from build123d import *

# Parameters (mm, degrees)
SKETCH1_W           = 23.2
SKETCH1_H           = 12.1
BOSS_EXTRUDE1_DEPTH = 21.6
BOSS_EXTRUDE2_DEPTH = 1.8
SKETCH5_R           = 6.05
BOSS_EXTRUDE3_DEPTH = 3.9
SKETCH6_R           = 2.345
BOSS_EXTRUDE4_DEPTH = 3.1
SKETCH7_W           = 3.926136304
SKETCH7_H           = 5.6
BOSS_EXTRUDE5_DEPTH = 3.3


with BuildPart() as part:
    # Sketch1 → Boss-Extrude1 (new body)
    with BuildSketch(Plane(origin=(0, 0, 0), x_dir=(1, 0, 0), z_dir=(0, 1, 0))):
        Rectangle(SKETCH1_W, SKETCH1_H)
    extrude(amount=BOSS_EXTRUDE1_DEPTH)

    # Sketch3 → Boss-Extrude2 (add)
    with BuildSketch(Plane(origin=(0, 15.5, 0), x_dir=(-1, 0, 0), z_dir=(0, -1, 0))):
        with BuildLine():
            Line((-11.6, 2.8e-08), (-11.6, 6.05))
            Line((-11.6, 6.05), (-16.1, 6.05))
            Line((-16.1, 6.05), (-16.1, 1.6))
            ThreePointArc((-16.1, 1.6), (-13.285381067, 2.387990792), (-11.6, 2.8e-08))
        make_face()
        with BuildLine():
            Line((-11.6, -6.05), (-11.6, 2.8e-08))
            ThreePointArc((-11.6, 2.8e-08), (-13.28538104, -2.387990782), (-16.1, -1.6))
            Line((-16.1, -1.6), (-16.1, -6.05))
            Line((-16.1, -6.05), (-11.6, -6.05))
        make_face()
        with BuildLine():
            ThreePointArc((16.1, -1.6), (13.285381054, -2.387990787), (11.6, -1e-09))
            Line((11.6, -1e-09), (11.6, -6.05))
            Line((11.6, -6.05), (16.1, -6.05))
            Line((16.1, -6.05), (16.1, -1.6))
        make_face()
        with BuildLine():
            Line((16.1, 1.6), (16.1, 6.05))
            Line((16.1, 6.05), (11.6, 6.05))
            Line((11.6, 6.05), (11.6, -1e-09))
            ThreePointArc((11.6, -1e-09), (13.285381053, 2.387990787), (16.1, 1.6))
        make_face()
    extrude(amount=-BOSS_EXTRUDE2_DEPTH)

    # Sketch5 → Boss-Extrude3 (add)
    with BuildSketch(Plane(origin=(0, 21.6, 0), x_dir=(1, 0, 0), z_dir=(0, 1, 0))):
        with Locations((5.55, 0)):
            Circle(SKETCH5_R)
    extrude(amount=BOSS_EXTRUDE3_DEPTH)

    # Sketch6 → Boss-Extrude4 (add)
    with BuildSketch(Plane(origin=(0, 25.5, 0), x_dir=(1, 0, 0), z_dir=(0, 1, 0))):
        with Locations((5.55, 0)):
            Circle(SKETCH6_R)
    extrude(amount=BOSS_EXTRUDE4_DEPTH)

    # Sketch7 → Boss-Extrude5 (add)
    with BuildSketch(Plane(origin=(0, 21.6, 0), x_dir=(1, 0, 0), z_dir=(0, 1, 0))):
        with Locations((-0.95, 0)):
            Rectangle(SKETCH7_W, SKETCH7_H)
    extrude(amount=BOSS_EXTRUDE5_DEPTH)


solid = part.part
Input: part model. Units: mm. Frame: model coordinates. A direction names the side the tool comes from. Give positions to 0.01 mm unless a question says otherwise; leave off trailing zeros. Write each loop counter-clockwise with the first axis right and the second up, starting at its lowest first coordinate (ties: lowest second). Pieces come first, ordered by that corner, then holes. Notation, with made-up numbers: M 8,-12.5 L 35,-12.5 A17 cw 35,7.5 Z; hole C 67,-16.75 d4. An arc over 180 degrees is marked long. Write item = value, one per line. Start each with the question number.
1) Reachability of faces 1 (the flat face through (10, 21.6, 5)), 2 (the flat face through (5, 25.5, 3)), 3 (the flat face through (-1, 23, -2.8)), 4 (the flat face through (-14, 17.3, -4)) from +Z, -Z, +X, -X, +Y, -Y: full face, straight path, thin tool, end or side. Return the list, or none.
2) Cut plane A-A on y = 16. Return the cut outline in (x, z), then the cut area to 3 significant figures.
3) Cut plane C-C on z = 3.5. Return the cut outline in (x, y).
4) Cut plane D-D on y = 22. Return the cut outline in (x, z).
5) Cut plane B-B on z = 1. Return the cut outline in (x, y).
6) First-contact query: pin 1 Ø2.5 at (x, z) = (-15, 2) entering from -Y; pin 2 Ø3.5 at (y, z) = (22.5, -0.5) entering from -X; pin 3 Ø1.6 at (x, y) = (-2, 23.5) entering from +Z; pin 4 Ø1 at (x, z) = (-12.5, 0.5) entering from +Y. Flat tips, straight axial feed; report the tip coordinate or a pass-through.
7) Material intervals for line 1 along Y through (x, z) = (-6, 1.5); line 2 along Y through (x, z) = (15, -5); line 3 along X through (y, z) = (18.25, -2.25), sorted ascending. Write a range as [from, to].
Solved:
q1.face_1 = +Z, +X, +Y
q1.face_2 = +Y
q1.face_3 = -Z, -X, +Y
q1.face_4 = +Z, -Z, -X, +Y
q2.outline = M -16.1,-6.05 L 16.1,-6.05 L 16.1,-1.6 A2.53 cw long 16.1,1.6 L 16.1,6.05 L -16.1,6.05 L -16.1,1.6 A2.53 cw long -16.1,-1.6 Z
q2.area = 352 mm2
q3.outline = M -16.1,15.5 L -11.6,15.5 L -11.6,0 L 11.6,0 L 11.6,15.5 L 16.1,15.5 L 16.1,17.3 L 11.6,17.3 L 11.6,21.6 L 10.48,21.6 L 10.48,25.5 L 0.62,25.5 L 0.62,21.6 L -11.6,21.6 L -11.6,17.3 L -16.1,17.3 Z
q4.outline = M -2.91,-2.8 L 0.19,-2.8 A6.05 ccw long 0.19,2.8 L -2.91,2.8 Z
q5.outline = M -11.81,15.5 L -11.6,15.5 L -11.6,0 L 11.6,0 L 11.6,15.5 L 11.81,15.5 L 11.81,17.3 L 11.6,17.3 L 11.6,21.6 L 11.52,21.6 L 11.52,25.5 L 7.67,25.5 L 7.67,28.6 L 3.43,28.6 L 3.43,25.5 L -0.42,25.5 L -0.42,24.9 L -2.91,24.9 L -2.91,21.6 L -11.6,21.6 L -11.6,17.3 L -11.81,17.3 Z
q6.pin_1 = 15.5
q6.pin_2 = -11.6
q6.pin_3 = 2.8
q6.pin_4 = through
q7.line_1 = [0, 21.6]
q7.line_2 = [15.5, 17.3]
q7.line_3 = [-11.6, 11.6]
